```python
from build123d import *

# Parameters (mm, degrees)
SKETCH_1_R               = 51
EXTRUDE_1_DEPTH          = 28
SKETCH_2_R               = 22.5
EXTRUDE_2_DEPTH          = 1
EXTRUDE_START            = 1
SKETCH_3_R               = 22.5
EXTRUDE_3_DEPTH          = 1
CUT_EXTRUDE_1_REACH      = 80.115
CUT_EXTRUDE_2_REACH      = 79.737
PATTERN_CIRCULAR_1_COUNT = 32


with BuildPart() as part:
    # 草图1 → 凸台-拉伸1 (new body)
    with BuildSketch(Plane.XY):
        Circle(SKETCH_1_R)
    extrude(amount=EXTRUDE_1_DEPTH)

    # 草图2 → 凸台-拉伸2 (add)
    with BuildSketch(Plane(origin=(0, 0, 0), x_dir=(-1, 0, 0), z_dir=(0, 0, -1))):
        with Locations(Location((0, 0, 0), (0, 0, 180))):
            Circle(SKETCH_2_R)
    extrude(amount=EXTRUDE_2_DEPTH)

    # 草图3 → 凸台-拉伸3 (add)
    with BuildSketch(Plane.XY.offset(28).offset(EXTRUDE_START)):
        Circle(SKETCH_3_R)
    extrude(amount=-EXTRUDE_3_DEPTH)

    # 草图4 → 切除-拉伸1 (cut, up to next)
    with BuildSketch(Plane(origin=(0, 0, -1), x_dir=(-1, 0, 0), z_dir=(0, 0, -1)), mode=Mode.PRIVATE) as cut_extrude_1_sk1:
        with BuildLine():
            Line((-4, 18.3), (-4, 14.456832295))
            ThreePointArc((-4, 14.456832295), (0, -15), (4, 14.456832295))
            Line((4, 14.456832295), (4, 18.3))
            Line((4, 18.3), (-4, 18.3))
        make_face()
    cut_extrude_1_tool1 = extrude(cut_extrude_1_sk1.sketch, amount=-CUT_EXTRUDE_1_REACH, mode=Mode.PRIVATE) & part.part
    add(cut_extrude_1_tool1.solids().sort_by_distance((0, 0.627325, -1))[0], mode=Mode.SUBTRACT)

    # 草图5 → 切除-拉伸2 (cut, up to next)
    with BuildSketch(Plane(origin=(0, 0, 0), x_dir=(-1, 0, 0), z_dir=(0, 0, -1)), mode=Mode.PRIVATE) as cut_extrude_2_sk1:
        with BuildLine():
            Line((-4, 50.842895276), (-1.859372488, 44.961569523))
            ThreePointArc((-1.859372488, 44.961569523), (0, 45), (1.859372488, 44.961569523))
            Line((1.859372488, 44.961569523), (4, 50.842895276))
            ThreePointArc((4, 50.842895276), (0, 51), (-4, 50.842895276))
        make_face()
    cut_extrude_2_tool1 = extrude(cut_extrude_2_sk1.sketch, amount=-CUT_EXTRUDE_2_REACH, mode=Mode.PRIVATE) & part.part
    cut_extrude_2 = cut_extrude_2_tool1.solids().sort_by_distance((0, 48.332211, 0))[0]
    add(cut_extrude_2, mode=Mode.SUBTRACT)

    # 阵列(圆周)1: 切除-拉伸2 ×32 about axis
    pattern_circular_1_axis = Axis((0, 0, 0), (0, 0, 1))
    for i in range(1, PATTERN_CIRCULAR_1_COUNT):
        add(cut_extrude_2.rotate(pattern_circular_1_axis, i * 360 / PATTERN_CIRCULAR_1_COUNT), mode=Mode.SUBTRACT)


solid = part.part
```
Design review of the part built by this model. Coordinates are the model's own, in mm. A direction names the side the tool comes from. Coordinates: 2 decimals unless noted, no trailing zeros. Order: outer loops, then holes, each group sorted by start corner. A loop starts at its lowest first (then second) coordinate and runs counter-clockwise, first axis right, second up. Notation, with made-up numbers: M 63,-23.5 L 104,-23.5 A19 ccw 104,4.5 Z; hole C 25,55.5 d6. An arc over 180 degrees is marked long. Answer as a JSON object with one key per item and string values. Group by question number.
1) Wall thickness on L1, parallel to X at y = 0, z = 15.75; L2, parallel to X at y = 39.5, z = 21.5; L3, parallel to Y at x = 38, z = 3.25: over which ranges is each line inside the solid? List them lowest first.
2) Mouldability with a two-part tool opening along X and no side actions: class faces 4 (the cylindrical face through (-45, 0, 14)), 5 (the flat face through (4, 16, 14)), 6 (the flat face through (31.819, -35.983, 13.804)) as pulls with the +X half, pulls with the -X half, needs draft (parallel to the pull), parting line crosses it, or undercut.
3) For pin 1 (1 mm diameter, centred on x = 39.5, z = 20, fed in from +Y); pin 2 (6 mm diameter, centred on x = 23, z = 12, fed in from +Y); pin 3 (3 mm diameter, centred on x = 32, y = -13, fed in from +Z); pin 4 (10 mm diameter, centred on y = 8.5, z = 12, fed in from +X), all flat-tipped, find the tip position at first contact; note any pin that passes through.
4) Add section B-B, the plane x = 0. Write out the cut boundary in (y, z), then the cut area to 3 significant figures.
5) Tool access review of faces 1 (the flat face through (-31.78, -35.9, 13.8)), 2 (the cylindrical face through (31.84, 31.8, 13.8)), 3 (the flat face through (21.008, -43.102, 13.804)): name each direction out of +Z, -Z, +X, -X, +Y, -Y from which nothing blocks a thin tool from reaching the whole face with its end or side.
6) Add section A-A, the plane y = 0. Write out the cut boundary in (x, z).
Computed values:
{
 "1": {"L1": "x = -45 to -15, 15 to 45", "L2": "x = -32.26 to -30.82, -23.7 to 23.7, 30.82 to 32.26", "L3": "y = -32.76 to -28.77, -24.1 to 24.1, 28.77 to 32.76"},
 "2": {"face 4": "pulls with the -X half", "face 5": "undercut", "face 6": "pulls with the +X half"},
 "3": {"pin 1": "stops at y = 32.86", "pin 2": "stops at y = 45.44", "pin 3": "stops at z = 28", "pin 4": "stops at x = 50.84"},
 "4": {"outline": "M -45,0 L -22.5,0 L -22.5,-1 L -15,-1 L -15,29 L -22.5,29 L -22.5,28 L -45,28 Z; M 18.3,-1 L 22.5,-1 L 22.5,0 L 45,0 L 45,28 L 22.5,28 L 22.5,29 L 18.3,29 Z", "area": "1,610 mm^2"},
 "5": {"face 1": "+Z, -Z, -X", "face 2": "+Z, -Z", "face 3": "+Z, -Z, -Y"},
 "6": {"outline": "M -45,0 L -22.5,0 L -22.5,-1 L -15,-1 L -15,29 L -22.5,29 L -22.5,28 L -45,28 Z; M 15,-1 L 22.5,-1 L 22.5,0 L 45,0 L 45,28 L 22.5,28 L 22.5,29 L 15,29 Z"}
}
